Design review of the part built by this model. Coordinates are the model's own, in mm. Give positions to 0.01 mm unless a question says otherwise; leave off trailing zeros. Write each loop counter-clockwise with the first axis right and the second up, starting at its lowest first coordinate (ties: lowest second). Pieces come first, ordered by that corner, then holes. Notation, with made-up numbers: M 62.25,87 L 70.25,87 A31 ccw 70.25,117 Z; hole C -28,-20.5 d6. An arc over 180 degrees is marked long. Use a Markdown table: item, result. Add a question column.
Autodesk Inventor part; units mm, degrees
ref_plane "YZ Plane" through (0, 0, 0) normal (1, 0, 0) x (0, 1, 0)
ref_plane "XZ Plane" through (0, 0, 0) normal (0, 1, 0) x (-1, 0, 0)
ref_plane "XY Plane" through (0, 0, 0) normal (0, 0, 1) x (1, 0, 0)
sketch "Sketch1" plane through (0, 0, 0) normal (0, 1, 0) x (-1, 0, 0)
  line L0 (0, 0) -> (250, 0)
  line L1 (250, 0) -> (250, -170)
  line L2 (250, -170) -> (0, -170)
  line L3 (0, -170) -> (0, 0)
  line L4 (0, 0) -> (150, 0)
  dimension "d0" = 250
  dimension "d1" = 170
  dimension "d2" = 150
extrude "Extrusion1" add sketch "Sketch1" along normal blind 10
sketch "Sketch2" plane through (0, 10, 0) normal (0, 1, 0) x (1, 0, 0)
  line L0 (0, 0) -> (-150, 0)
  line L1 (-250, 0) -> (0, 0)
  line L2 (0, 170) -> (-250, 170)
  circle A0 centre (-75, 85) radius 20
  dimension "d5" = 150
  dimension "d6" = 40
extrude "Extrusion2" cut sketch "Sketch2" against normal blind 10
sketch "Sketch3" plane through (0, 10, 0) normal (0, 1, 0) x (1, 0, 0)
  circle A0 centre (-75, 85) radius 20
  circle A1 centre (-75, 85) radius 23.5
  point P0 (0, 0)
  dimension "d9" = 47
extrude "Extrusion3" cut sketch "Sketch3" against normal blind 9
sketch "Sketch4" plane through (0, 10, 0) normal (0, 1, 0) x (1, 0, 0)
  circle A0 centre (-75, 85) radius 20
  circle A1 centre (-75, 85) radius 30
  circle A2 centre (-75, 85) radius 37.5
  point P0 (0, 0)
  dimension "d12" = 60
  dimension "d13" = 75
extrude "Extrusion4" add sketch "Sketch4" along normal blind 4 contours A2
sketch "Sketch5" plane through (0, 0, 0) normal (0, -1, 0) x (1, 0, 0)
  circle A0 centre (-75, -85) radius 20
  circle A1 centre (-75, -85) radius 20.5
  circle A2 centre (-75, -85) radius 20
  point P0 (0, 0)
  dimension "d16" = 41
  dimension "d17" = 40
extrude "Extrusion5" add sketch "Sketch5" along normal blind 2
sketch "Sketch6" plane through (0, 10, 0) normal (0, 1, 0) x (1, 0, 0)
  circle A0 centre (-75, 85) radius 23.5
  circle A1 centre (-75, 85) radius 50
  circle A2 centre (-230.6, 85) radius 10
  point P0 (0, 0)
  dimension "d20" = 100
  dimension "d22" = 20
extrude "Extrusion6" cut sketch "Sketch6" against normal blind 10 contours A2
sketch "Sketch7" plane through (0, 0, 0) normal (0, -1, 0) x (1, 0, 0)
  line L0 (-250, -170) -> (-250, 0)
  line L1 (-250, 0) -> (-320, 0)
  line L2 (-320, 0) -> (-320, -170)
  line L3 (-320, -170) -> (-250, -170)
  line L4 (-250, -170) -> (-250, 0)
  point P0 (0, 0)
  dimension "d25" = 70
  dimension "d26" = 170
extrude "Extrusion7" add sketch "Sketch7" against normal blind 10
properties part number "b_base cover_test 1"
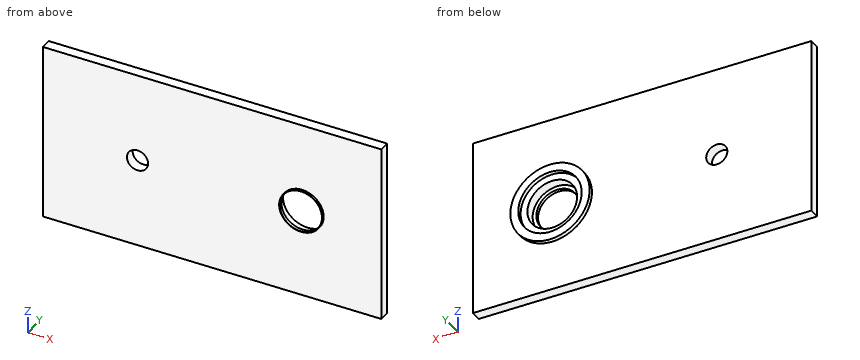
(1) Add section C-C on y = 6.5. Give the boundary of the cut face in (x, z), then the cut area to 3 significant figures.
(2) For pin 1 (2 mm diameter, centred on x = -245.5, z = -121, fed in from +Y); pin 2 (1 mm diameter, centred on x = -53, z = -36, fed in from -Y), all flat-tipped, find the tip position at first contact; note any pin that passes through.
(3) Wall thickness on L1, parallel to X at y = 0.1, z = -85; L2, parallel to Z at x = -230.6, y = 6.25; L3, parallel to Z at x = -75, y = 11.4: over which ranges is each line inside the solid? List them lowest first.
(4) Add section A-A on z = -85. Give the boundary of the cut face in (x, y), then the cut area to 3 significant figures.
(5) Add section D-D on x = -75. Give the boundary of the cut face in (y, z), then the cut area to 3 significant figures.
(6) Add section B-B on x = -230.6. Give the boundary of the cut face in (y, z), then the cut area to 3 significant figures.
From the geometry:
| question | item | result |
|---|---|---|
| 1 | outline | M -320,-170 L 0,-170 L 0,0 L -320,0 Z; hole C -230.6,-85 d20; hole C -75,-85 d47 |
| 1 | area | 52,400 mm^2 |
| 2 | pin 1 | stops at y = 10 |
| 2 | pin 2 | stops at y = 0 |
| 3 | L1 | x = -320 to -240.6, -220.6 to -95, -55 to 0 |
| 3 | L2 | z = -170 to -95, -75 to 0 |
| 3 | L3 | z = -122.5 to -115, -55 to -47.5 |
| 4 | outline | M -320,0 L -240.6,0 L -240.6,10 L -320,10 Z; M -220.6,0 L -95.5,0 L -95.5,-2 L -95,-2 L -95,1 L -98.5,1 L -98.5,10 L -105,10 L -105,14 L -112.5,14 L -112.5,10 L -220.6,10 Z; M -55,-2 L -54.5,-2 L -54.5,0 L 0,0 L 0,10 L -37.5,10 L -37.5,14 L -45,14 L -45,10 L -51.5,10 L -51.5,1 L -55,1 Z |
| 4 | area | 2,600 mm^2 |
| 5 | outline | M -2,-105.5 L 0,-105.5 L 0,-170 L 10,-170 L 10,-122.5 L 14,-122.5 L 14,-115 L 10,-115 L 10,-108.5 L 1,-108.5 L 1,-105 L -2,-105 Z; M -2,-65 L 1,-65 L 1,-61.5 L 10,-61.5 L 10,-55 L 14,-55 L 14,-47.5 L 10,-47.5 L 10,0 L 0,0 L 0,-64.5 L -2,-64.5 Z |
| 5 | area | 1,300 mm^2 |
| 6 | outline | M 0,-170 L 10,-170 L 10,-95 L 0,-95 Z; M 0,-75 L 10,-75 L 10,0 L 0,0 Z |
| 6 | area | 1,500 mm^2 |
